```python
from build123d import *

# Parameters (mm, degrees)
CROQUIS2_W                = 23.4
CROQUIS2_H                = 23.4
CROQUIS2_W_2              = 19.4
CROQUIS2_H_2              = 19.4
SALIENTE_EXTRUIR1_DEPTH   = 10
CROQUIS2_W_3              = 29.4
CROQUIS2_H_3              = 29.4
CROQUIS2_W_4              = 25.4
CROQUIS2_H_4              = 25.4
SALIENTE_EXTRUIR1_2_DEPTH = 10
CROQUIS3_W                = 29.4
CROQUIS3_H                = 29.4
CROQUIS3_W_2              = 19.4
CROQUIS3_H_2              = 19.4
SALIENTE_EXTRUIR2_DEPTH   = 2
CROQUIS4_W                = 26.4
CROQUIS4_H                = 26.4
CROQUIS4_W_2              = 22.4
CROQUIS4_H_2              = 22.4
CORTAR_EXTRUIR1_DEPTH     = 10


with BuildPart() as part:
    # Croquis2 → Saliente-Extruir1 (new body)
    with BuildSketch(Plane(origin=(0, 0, 0), x_dir=(0, 0, -1), z_dir=(1, 0, 0))):
        with Locations((-12.7, -12.7)):
            Rectangle(CROQUIS2_W, CROQUIS2_H)
        with Locations((-12.7, -12.7)):
            Rectangle(CROQUIS2_W_2, CROQUIS2_H_2, mode=Mode.SUBTRACT)
    extrude(amount=SALIENTE_EXTRUIR1_DEPTH)



with BuildPart() as body_2:
    # Croquis2 → Saliente-Extruir1 2 (new body)
    with BuildSketch(Plane(origin=(0, 0, 0), x_dir=(0, 0, -1), z_dir=(1, 0, 0))):
        with Locations((-12.7, -12.7)):
            Rectangle(CROQUIS2_W_3, CROQUIS2_H_3)
        with Locations((-12.7, -12.7)):
            Rectangle(CROQUIS2_W_4, CROQUIS2_H_4, mode=Mode.SUBTRACT)
    extrude(amount=SALIENTE_EXTRUIR1_2_DEPTH)


with BuildPart() as part_1:
    add(part.part)

    add(body_2.part)  # Saliente-Extruir2 merges body 2
    # Croquis3 → Saliente-Extruir2 (add)
    with BuildSketch(Plane.ZY):
        with Locations((12.7, -12.7)):
            Rectangle(CROQUIS3_W, CROQUIS3_H)
        with Locations((12.7, -12.7)):
            Rectangle(CROQUIS3_W_2, CROQUIS3_H_2, mode=Mode.SUBTRACT)
    extrude(amount=SALIENTE_EXTRUIR2_DEPTH)

    # Croquis4 → Cortar-Extruir1 (cut)
    with BuildSketch(Plane(origin=(10, 0, 0), x_dir=(0, 0, -1), z_dir=(1, 0, 0))):
        with Locations((-12.7, -12.7)):
            Rectangle(CROQUIS4_W, CROQUIS4_H)
        with Locations((-12.7, -12.7)):
            Rectangle(CROQUIS4_W_2, CROQUIS4_H_2, mode=Mode.SUBTRACT)
    extrude(amount=-CORTAR_EXTRUIR1_DEPTH, mode=Mode.SUBTRACT)


solid = part_1.part
```
The model under review builds one solid part; all positions refer to its coordinate system, in mm. A direction names the side the tool comes from. Coordinates: 2 decimals unless noted, no trailing zeros. Order: outer loops, then holes, each group sorted by start corner. A loop starts at its lowest first (then second) coordinate and runs counter-clockwise, first axis right, second up. Notation, with made-up numbers: (49.25, -18.75) -> (86.25, -18.75) arc R20 cw to (86.25, 2.25) -> close; hole circle Ø8 at (65, 47.25). An arc over 180 degrees is marked (long way). Answer in a Markdown table with one row per item. Add a question column.
Item 1: Machinability: for faces 1 (the flat face through (5, -13, 23.9)), 2 (the flat face through (-2, -2.7, 12.5)), 3 (the flat face through (4, -22.4, 13)), which of the approach directions +Z, -Z, +X, -X, +Y, -Y give a long, thin tool a straight path to every point of the face, cutting with its end or side? Answer none if there is none.
Item 2: To check wall thickness, follow probe 1 along Z at (x, y) = (1.25, -10.75); probe 2 along Y at (x, z) = (0.5, 18); probe 3 along Z at (x, y) = (9.25, -2). State the ranges of each line that lie inside material, in increasing order.
Item 3: We need section C-C on x = -1. Write out the cut boundary in (y, z).
Item 4: We need section A-A on x = 9. Write out the cut boundary in (y, z), plus the area to 3 significant figures.
Item 5: Mouldability with a two-part tool opening along Y and no side actions: class faces 4 (the flat face through (4, -13, 27.4)), 5 (the flat face through (5, -1.5, 13)) as +Y half, -Y half, draft (parallel to the pull), parting line (faces both ways), or undercut.
Item 6: We need section B-B on z = 12.5. Write out the cut boundary in (x, y), plus the area to 3 significant figures.
Item 7: We need section D-D on y = -24.5. Write out the cut boundary in (x, z), plus the area to 3 significant figures.
Final values:
| question | item | result |
|---|---|---|
| 1 | face 1 | +X |
| 1 | face 2 | +Z, -Z, -X, +Y, -Y |
| 1 | face 3 | +X, -X |
| 2 | probe 1 | z = -2 to -0.5, 1.5 to 3, 22.4 to 23.9, 25.9 to 27.4 |
| 2 | probe 2 | y = -27.4 to -25.9, -23.9 to -22.4, -3 to -1.5, 0.5 to 2 |
| 2 | probe 3 | z = -2 to -0.5, 1.5 to 23.9, 25.9 to 27.4 |
| 3 | outline | (-27.4, -2) -> (2, -2) -> (2, 27.4) -> (-27.4, 27.4) -> close; hole (-22.4, 3) -> (-3, 3) -> (-3, 22.4) -> (-22.4, 22.4) -> close |
| 4 | outline | (-27.4, -2) -> (2, -2) -> (2, 27.4) -> (-27.4, 27.4) -> close; (-23.9, 1.5) -> (-1.5, 1.5) -> (-1.5, 23.9) -> (-23.9, 23.9) -> close; hole (-25.9, -0.5) -> (0.5, -0.5) -> (0.5, 25.9) -> (-25.9, 25.9) -> close; hole (-22.4, 3) -> (-3, 3) -> (-3, 22.4) -> (-22.4, 22.4) -> close |
| 4 | area | 293 mm2 |
| 5 | face 4 | draft |
| 5 | face 5 | undercut |
| 6 | outline | (-2, -27.4) -> (10, -27.4) -> (10, -25.9) -> (0, -25.9) -> (0, -23.9) -> (10, -23.9) -> (10, -22.4) -> (-2, -22.4) -> close; (-2, -3) -> (10, -3) -> (10, -1.5) -> (0, -1.5) -> (0, 0.5) -> (10, 0.5) -> (10, 2) -> (-2, 2) -> close |
| 6 | area | 80.0 mm2 |
| 7 | outline | (-2, -2) -> (10, -2) -> (10, -0.5) -> (0, -0.5) -> (0, 25.9) -> (10, 25.9) -> (10, 27.4) -> (-2, 27.4) -> close |
| 7 | area | 88.8 mm2 |
